from build123d import *

# Parameters (mm, degrees)
SKETCH1_R           = 1.4
BOSS_EXTRUDE2_DEPTH = 4


with BuildPart() as part:
    # Sketch1 → Boss-Extrude2 (new body)
    with BuildSketch(Plane.XY):
        with BuildLine():
            Line((-0.000688459, -12.983908279), (-0.000688459, 65.016091721))
            ThreePointArc((-0.000688459, 65.016091721), (-6.500688459, 71.516091721), (-13.000688459, 65.016091721))
            Line((-13.000688459, 65.016091721), (-11.000688459, -12.983908279))
            ThreePointArc((-11.000688459, -12.983908279), (-5.500688459, -18.483908279), (-0.000688459, -12.983908279))
        make_face()
        with Locations((-6.500688459, 65.016091721)):
            Circle(SKETCH1_R, mode=Mode.SUBTRACT)
        with Locations((-5.500688459, -12.983908279)):
            Circle(SKETCH1_R, mode=Mode.SUBTRACT)
        with Locations((-6.012756351, 40.016091721)):
            Circle(SKETCH1_R, mode=Mode.SUBTRACT)
    extrude(amount=BOSS_EXTRUDE2_DEPTH)


solid = part.part
Verification items for the finished model (mm, model axes). Give positions to 0.01 mm unless a question says otherwise; leave off trailing zeros. Write each loop counter-clockwise with the first axis right and the second up, starting at its lowest first coordinate (ties: lowest second). Pieces come first, ordered by that corner, then holes. Notation, with made-up numbers: (46, 18) - (89, 18) arc R24 ccw to (89, 30) - close; hole circle Ø9 at (66, 89). An arc over 180 degrees is marked (long way). Answer as CSV lines item,"result". Start each with the question number.
1. Thickness scan on line 1 (Y direction, x = -7, z = 2.1); line 2 (Y direction, x = -6.25, z = 2.8); line 3 (Y direction, x = -6.75, z = 1.8). Record the ranges inside material, lowest first.
2. Sectioned sample at B-B (z = 2.75). Record the boundary of the cut face in (x, y).
3. Sectioned sample at C-C (x = -1.5). Record the boundary of the cut face in (y, z), then the cut area to 3 significant figures.
4. Depth check by flat-ended pin: pin 1 (3 mm diameter, centred on x = -6.5, y = 65.02, fed in from +Z); pin 2 (2 mm diameter, centred on y = 52, z = 1.5, fed in from -X); pin 3 (1.5 mm diameter, centred on x = -5.5, z = 0.5, fed in from +Y). Enter the tip coordinate at first touch or a pass-through.
5. Sectioned sample at A-A (x = -6). Record the boundary of the cut face in (y, z).
6. Draft check along X on faces 1 (the face through (-6.358, 71.515, 1.972)), 2 (the face through (-0.001, 25, 2)), 3 (the face through (-6.7, 66.4, 2)), 4 (the face through (-7, 27, 4)). Enter one of: pulls with the +X half, pulls with the -X half, needs draft (parallel to the pull), parting line crosses it, or undercut.
7. Sectioned sample at D-D (y = 32.5). Record the boundary of the cut face in (x, z).
Derived:
1,line 1,"-18.28 to 39.02, 41.01 to 63.71, 66.32 to 71.5"
1,line 2,"-18.43 to -14.17, -11.8 to 38.64, 41.4 to 63.64, 66.39 to 71.51"
1,line 3,"-18.34 to -13.62, -12.35 to 38.83, 41.21 to 63.64, 66.39 to 71.51"
2,outline,"(-13, 65.02) - (-11, -12.98) arc R5.5 ccw to (0, -12.98) - (0, 65.02) arc R6.5 ccw to start; hole circle Ø2.8 at (-6.5, 65.02); hole circle Ø2.8 at (-6.01, 40.02); hole circle Ø2.8 at (-5.5, -12.98)"
3,outline,"(-16.76, 0) - (69.17, 0) - (69.17, 4) - (-16.76, 4) - close"
3,area,"344 mm²"
4,pin 1,"z = 4"
4,pin 2,"x = -12.69"
4,pin 3,"y = 71.51"
5,outline,"(-18.46, 0) - (-14.29, 0) - (-14.29, 4) - (-18.46, 4) - close; (-11.68, 0) - (38.62, 0) - (38.62, 4) - (-11.68, 4) - close; (41.42, 0) - (63.71, 0) - (63.71, 4) - (41.42, 4) - close; (66.32, 0) - (71.5, 0) - (71.5, 4) - (66.32, 4) - close"
6,face 1,"parting line crosses it"
6,face 2,"pulls with the +X half"
6,face 3,"undercut"
6,face 4,"needs draft"
7,outline,"(-12.17, 0) - (0, 0) - (0, 4) - (-12.17, 4) - close"
